from build123d import *

# Parameters (mm, degrees)
BOSS_EXTRUDE1_DEPTH = 40
SKETCH3_W           = 11.5
SKETCH3_H           = 44
CUT_EXTRUDE1_DEPTH  = 30
SKETCH4_W           = 30.254833929
SKETCH4_H           = 40
CUT_EXTRUDE2_DEPTH  = 13.45
SKETCH5_W           = 32
SKETCH5_H           = 40
CUT_EXTRUDE3_DEPTH  = 13.45
SKETCH6_R           = 2.5
CUT_EXTRUDE4_DEPTH  = 100
CUT_EXTRUDE5_DEPTH  = 28.12


with BuildPart() as part:
    # Sketch1 → Boss-Extrude1 (new body)
    with BuildSketch(Plane.XY):
        Polygon((0, 0), (-70, 0), (-70, -70), (-30, -70), (-30, -40), (0, -40), align=None)
    extrude(amount=BOSS_EXTRUDE1_DEPTH)

    # Sketch3 → Cut-Extrude1 (cut)
    with BuildSketch(Plane.ZY.offset(70)):
        with Locations((14.25, -35.45)):
            Rectangle(SKETCH3_W, SKETCH3_H)
        with Locations((25.75, -35.45)):
            Rectangle(SKETCH3_W, SKETCH3_H)
    extrude(amount=-CUT_EXTRUDE1_DEPTH, mode=Mode.SUBTRACT)

    # Sketch4 → Cut-Extrude2 (cut)
    with BuildSketch(Plane(origin=(0, 0, 0), x_dir=(1, 0, 0), z_dir=(0, 1, 0))):
        with Locations((-46.872583036, -20)):
            Rectangle(SKETCH4_W, SKETCH4_H)
    extrude(amount=-CUT_EXTRUDE2_DEPTH, mode=Mode.SUBTRACT)

    # Sketch5 → Cut-Extrude3 (cut)
    with BuildSketch(Plane.XZ.offset(70)):
        with Locations((-46, 20)):
            Rectangle(SKETCH5_W, SKETCH5_H)
    extrude(amount=-CUT_EXTRUDE3_DEPTH, mode=Mode.SUBTRACT)

    # Sketch6 → Cut-Extrude4 (cut)
    with BuildSketch(Plane.ZY.offset(70)):
        with Locations((15, -10.4)):
            Circle(SKETCH6_R)
        with Locations((25, -10.4)):
            Circle(SKETCH6_R)
        with Locations((25, -60.5)):
            Circle(SKETCH6_R)
        with Locations((15, -60.5)):
            Circle(SKETCH6_R)
    extrude(amount=-CUT_EXTRUDE4_DEPTH, mode=Mode.SUBTRACT)

    # Sketch7 → Cut-Extrude5 (cut)
    with BuildSketch(Plane(origin=(0, 0, 0), x_dir=(0, 0, -1), z_dir=(1, 0, 0))):
        with BuildLine():
            ThreePointArc((-31, -24.34), (-20, -35.34), (-9, -24.34))
            Line((-9, -24.34), (-31, -24.34))
        make_face()
        with BuildLine():
            Line((-31, -24.34), (-9, -24.34))
            ThreePointArc((-9, -24.34), (-20, -13.34), (-31, -24.34))
        make_face()
    extrude(amount=-CUT_EXTRUDE5_DEPTH, mode=Mode.SUBTRACT)


solid = part.part
Input: part model. Units: mm. Frame: model coordinates. A direction names the side the tool comes from. Give positions to 0.01 mm unless a question says otherwise; leave off trailing zeros. Write each loop counter-clockwise with the first axis right and the second up, starting at its lowest first coordinate (ties: lowest second). Pieces come first, ordered by that corner, then holes.
Q1. Section D-D, the plane y = -10.4. Output: boundary loops of the cut face in (x, z), plus the area to 3 significant figures.
Q2. Section A-A, the plane x = -56. Output: boundary loops of the cut face in (y, z).
Q3. First-contact query: P1, Ø11, axis at y = -22, z = 16.5, coming from the +X side; P2, Ø24, axis at x = -45.5, z = 17.5, coming from the +Y side; P3, Ø3, axis at y = -41, z = 29, coming from the -X side. Flat tips, straight axial feed; report the tip coordinate or a pass-through.
Q4. Section B-B, the plane y = -60.5. Output: boundary loops of the cut face in (x, z).
Q5. Section C-C, the plane z = 20. Output: boundary loops of the cut face in (x, y).
Q6. Set-up query: faces 1 (the face through (-28.12, -24, 20)), 2 (the face through (-66, -57.45, 20)), 3 (the face through (-39, -56.55, 20)), 4 (the face through (-37, -13.45, 20)), 5 (the face through (-55, -36, 31.5)). Return all of +Z, -Z, +X, -X, +Y, -Y with unobstructed straight access to the full face (end or side cutting, diameter ignored); none if empty.
Q7. Pull-direction query (Z, two-part tool) for faces 6 (the face through (-66, -70, 20)), 7 (the face through (-35, -27, 40)), 8 (the face through (-16.1, -10.3, 12.5)); classes: pulls with the +Z half, pulls with the -Z half, needs draft (parallel to the pull), parting line crosses it, or undercut.
Q8. Material intervals for probe 1 along Y at (x, z) = (-68, 25); probe 2 along Z at (x, y) = (-43, -31), sorted ascending.
Filled in:
1. outline: (-70, 0) - (-62, 0) - (-62, 12.5) - (-70, 12.5) - close; (-70, 17.5) - (-62, 17.5) - (-62, 22.5) - (-70, 22.5) - close; (-70, 27.5) - (-62, 27.5) - (-62, 40) - (-70, 40) - close; (-31.75, 0) - (0, 0) - (0, 12.5) - (-31.75, 12.5) - close; (-31.75, 17.5) - (0, 17.5) - (0, 22.5) - (-31.75, 22.5) - close; (-31.75, 27.5) - (0, 27.5) - (0, 40) - (-31.75, 40) - close
1. area: 1,190 mm2
2. outline: (-56.55, 0) - (-13.45, 0) - (-13.45, 8.5) - (-56.55, 8.5) - close; (-56.55, 31.5) - (-13.45, 31.5) - (-13.45, 40) - (-56.55, 40) - close
3. P1: stops at x = -28.12
3. P2: stops at y = -13.45
3. P3: stops at x = -40
4. outline: (-70, 0) - (-62, 0) - (-62, 12.5) - (-70, 12.5) - close; (-70, 17.5) - (-62, 17.5) - (-62, 22.5) - (-70, 22.5) - close; (-70, 27.5) - (-62, 27.5) - (-62, 40) - (-70, 40) - close
5. outline: (-70, -70) - (-62, -70) - (-62, -57.45) - (-70, -57.45) - close; (-70, -13.45) - (-62, -13.45) - (-62, 0) - (-70, 0) - close; (-40, -56.55) - (-30, -56.55) - (-30, -40) - (0, -40) - (0, -35.34) - (-28.12, -35.34) - (-28.12, -13.34) - (0, -13.34) - (0, 0) - (-31.75, 0) - (-31.75, -13.45) - (-40, -13.45) - close
6. face 1: +X
6. face 2: +X, -X
6. face 3: +Z, -Z, +X, -Y
6. face 4: +Z, -Z, +Y
6. face 5: -X
7. face 6: needs draft
7. face 7: pulls with the +Z half
7. face 8: undercut
8. probe 1: y = -70 to -63, -58 to -57.45, -13.45 to -12.9, -7.9 to 0
8. probe 2: z = 0 to 8.5, 31.5 to 40
